```python
from build123d import *

# Parameters (mm, degrees)
EXTRUSION1_DEPTH = 11
EXTRUSION3_DEPTH = 186
EXTRUSION4_DEPTH = 12
EXTRUSION5_DEPTH = 2
CONG_1_R         = 2
ESQUISSE6_R      = 1.75
EXTRUSION6_DEPTH = 40


with BuildPart() as part:
    # Esquisse1 → Extrusion1 (new body)
    with BuildSketch(Plane(origin=(0, 0, 0), x_dir=(1, 0, 0), z_dir=(0, 1, 0))):
        with BuildLine():
            Line((0, 0), (22, 0))
            ThreePointArc((22, 0), (34.5, 12.5), (22, 25))
            Line((22, 25), (0, 25))
            ThreePointArc((0, 25), (-12.5, 12.5), (0, 0))
        make_face()
    extrude(amount=EXTRUSION1_DEPTH)

    # Esquisse3 → Extrusion3 (add)
    with BuildSketch(Plane(origin=(0, 11, 0), x_dir=(1, 0, 0), z_dir=(0, 1, 0))):
        with BuildLine():
            Line((0, 1), (22, 1))
            ThreePointArc((22, 1), (33.5, 12.5), (22, 24))
            Line((22, 24), (0, 24))
            ThreePointArc((0, 24), (-11.5, 12.5), (0, 1))
        make_face()
    extrude(amount=EXTRUSION3_DEPTH)

    # Esquisse4 → Extrusion4 (add)
    with BuildSketch(Plane(origin=(0, 197, 0), x_dir=(1, 0, 0), z_dir=(0, 1, 0))):
        with BuildLine():
            Line((0, 25), (22, 25))
            ThreePointArc((22, 25), (34.5, 12.5), (22, 0))
            Line((22, 0), (0, 0))
            ThreePointArc((0, 0), (-12.5, 12.5), (0, 25))
        make_face()
    extrude(amount=EXTRUSION4_DEPTH)

    # Esquisse5 → Extrusion5 (add)
    with BuildSketch(Plane(origin=(0, 209, 0), x_dir=(1, 0, 0), z_dir=(0, 1, 0))):
        with BuildLine():
            Line((0, 17.5), (22, 17.5))
            ThreePointArc((22, 17.5), (27, 12.5), (22, 7.5))
            Line((22, 7.5), (0, 7.5))
            ThreePointArc((0, 7.5), (-5, 12.5), (0, 17.5))
        make_face()
    extrude(amount=EXTRUSION5_DEPTH)

    # Congé1
    cong_1_edges = [part.edges().sort_by_distance(p)[0] for p in [
        (-12.5, 209, -12.5),
        (11, 209, 0),
        (34.5, 209, -12.5),
        (11, 209, -25),
        (11, 0, -25),
        (34.5, 0, -12.5),
        (11, 0, 0),
        (-12.5, 0, -12.5),
    ]]
    fillet(cong_1_edges, radius=CONG_1_R)

    # Esquisse6 → Extrusion6 (add)
    with BuildSketch(Plane(origin=(0, 211, 0), x_dir=(1, 0, 0), z_dir=(0, 1, 0))):
        with Locations((9.1, 12.5)):
            Circle(ESQUISSE6_R)
        with Locations((12.9, 12.5)):
            Circle(ESQUISSE6_R)
    extrude(amount=EXTRUSION6_DEPTH)


solid = part.part
```
Geometry check sheet. Reference: the model listing, model coordinates, mm. A direction names the side the tool comes from. Round coordinates to 2 decimals unless told otherwise and drop trailing zeros. Order: outer loops, then holes, each group sorted by start corner. A loop starts at its lowest first (then second) coordinate and runs counter-clockwise, first axis right, second up. Notation, with made-up numbers: M 28.5,-31 L 36.5,-31 A7 ccw 36.5,-27 Z; hole C 62.25,44.25 d1. An arc over 180 degrees is marked long. Answer as CSV lines item,"result".
1) Tool access check on faces 5 (the face through (33.497, 102.698, -12.247)), 6 (the face through (10.9, 11, -24.6)), 7 (the face through (27, 210, -12.6)), 8 (the face through (11, 103, -24)). Record the directions out of +Z, -Z, +X, -X, +Y, -Y that give a thin tool (end or side, any length) a straight path to the whole face; none if there is none.
Entries:
face 5,"+X"
face 6,"none"
face 7,"+X, +Y"
face 8,"-Z, +X, -X"
2) Thickness scan on probe 1 along Z at (x, y) = (-1, 153.5); probe 2 along Y at (x, z) = (22, -4.5); probe 3 along X at (y, z) = (117.5, -12.5). Record the ranges inside material, lowest first. Write a range as [from, to].
Entries:
probe 1,"[-23.96, -1.04]"
probe 2,"[0, 209]"
probe 3,"[-11.5, 33.5]"
3) Sectioned sample at A-A on y = 214. Record the cut outline in (x, z), and give its area (3 significant figures).
Entries:
outline,"C 9.1,-12.5 d3.5; C 12.9,-12.5 d3.5"
area,"19.2 mm2"
4) Sectioned sample at B-B on y = 68.5. Record the cut outline in (x, z).
Entries:
outline,"M 0,-24 L 22,-24 A11.5 ccw 22,-1 L 0,-1 A11.5 ccw Z"
5) Gauge pin test, flat ends, axial feed: pin 1 Ø2 at (x, z) = (3.5, -8) entering from +Y; pin 2 Ø10 at (x, y) = (21, 86) entering from -Z; pin 3 Ø1 at (x, y) = (15.5, 27) entering from +Z. Record the tip position at first contact, or that the pin passes through.
Entries:
pin 1,"y = 211"
pin 2,"z = -24"
pin 3,"z = -1"
6) Mould release check, pull along Y, two halves, no side actions. Record for faces 1 (the face through (34.497, 6.437, -12.225)), 2 (the face through (11, 103, -1)), 3 (the face through (11, 211, -11)), 4 (the face through (11, 0, -13)): +Y half, -Y half, draft (parallel to the pull), parting line (faces both ways), or undercut.
Entries:
face 1,"draft"
face 2,"undercut"
face 3,"+Y half"
face 4,"-Y half"
